Build history of the part. All positions in model axes, mm. A direction names the side the tool comes from. Round coordinates to 2 decimals unless told otherwise and drop trailing zeros. Loops run counter-clockwise (first coordinate to the right, second up) from the corner with the lowest first, then second, coordinate; pieces in that order, holes last.
from build123d import *

# Parameters (mm, degrees)
F0_R      = 20
F1_DEPTH  = 4
F2_R      = 9
F2_R_2    = 5.1
F3_DEPTH  = 20
F5_DEPTH  = 10
F6_W      = 5.5
F6_H      = 1.8
F7_DEPTH  = 5.5
F8_R      = 1.5
F9_DEPTH  = 11
F10_SIZE  = 5.99999
F12_DEPTH = 25


# Not quite as in the source:
# - a fillet or chamfer is up to 0.001 mm smaller than in the source, because OpenCascade refuses the exact size


with BuildPart() as f1:
    # F0 (on Top) → F1 (new body)
    with BuildSketch(Plane.XY):
        Circle(F0_R)
    extrude(amount=F1_DEPTH)

    # F2 (on face) → F3 (join)
    with BuildSketch(Plane.XY.offset(4)):
        Circle(F2_R)
        Circle(F2_R_2, mode=Mode.SUBTRACT)
    extrude(amount=F3_DEPTH)

    # F4 (on face) → F5 (join)
    with BuildSketch(Plane.XY.offset(4)):
        with BuildLine():
            Line((-3.5, 15), (-3.5, 8.2915619759))
            ThreePointArc((-3.5, 8.2915619759), (0, 9), (3.5, 8.2915619759))
            Line((3.5, 8.2915619759), (3.5, 15))
            Line((3.5, 15), (-3.5, 15))
        make_face()
        with BuildLine():
            Line((15, 3.5), (8.2915619759, 3.5))
            ThreePointArc((8.2915619759, 3.5), (8.8211126788, 1.785489039), (9, 0))
            ThreePointArc((9, 0), (8.8211126788, -1.785489039), (8.2915619759, -3.5))
            Line((8.2915619759, -3.5), (15, -3.5))
            Line((15, -3.5), (15, 3.5))
        make_face()
        with BuildLine():
            Line((-8.2915619759, 3.5), (-15, 3.5))
            Line((-15, 3.5), (-15, -3.5))
            Line((-15, -3.5), (-8.2915619759, -3.5))
            ThreePointArc((-8.2915619759, -3.5), (-9, 0), (-8.2915619759, 3.5))
        make_face()
        with BuildLine():
            ThreePointArc((3.5, -8.2915619759), (0, -9), (-3.5, -8.2915619759))
            Line((-3.5, -8.2915619759), (-3.5, -15))
            Line((-3.5, -15), (3.5, -15))
            Line((3.5, -15), (3.5, -8.2915619759))
        make_face()
    extrude(amount=F5_DEPTH)

    # F6 (on face) → F7 (cut)
    with BuildSketch(Plane.XY.offset(14)):
        with Locations((0, -11.6)):
            Rectangle(F6_W, F6_H)
    extrude(amount=-F7_DEPTH, mode=Mode.SUBTRACT)

    # F8 (on face) → F9 (cut)
    with BuildSketch(Plane.XZ.offset(15)):
        with Locations((0, 11.25)):
            Circle(F8_R)
    extrude(amount=-F9_DEPTH, mode=Mode.SUBTRACT)

    # F10 (size 6 in the source; OpenCascade refuses exactly that, so slightly less here)
    f10_edges = [f1.edges().sort_by_distance(p)[0] for p in [
        (15, 0, 14),
        (0, 15, 14),
        (-15, 0, 14),
    ]]
    chamfer(f10_edges, length=F10_SIZE)

    # F11 (on face) → F12 (cut)
    with BuildSketch(Plane(origin=(0, 0, 0), x_dir=(1, 0, 0), z_dir=(0, 0, -1))):
        with BuildLine():
            ThreePointArc((-10.6066017178, 10.6066017178), (-9.8758984631, 11.2901120254), (-9.1012534477, 11.9233881795))
            ThreePointArc((-9.1012534477, 11.9233881795), (-12.0208152802, 12.0208152802), (-11.9233881795, 9.1012534477))
            ThreePointArc((-11.9233881795, 9.1012534477), (-11.2901120254, 9.8758984631), (-10.6066017178, 10.6066017178))
        make_face()
        with BuildLine():
            Line((-10.6066017178, 10.6066017178), (-9.1923881554, 9.1923881554))
            ThreePointArc((-9.1923881554, 9.1923881554), (-8.7588426528, 9.8412348531), (-8.6066017178, 10.6066017178))
            ThreePointArc((-8.6066017178, 10.6066017178), (-8.7343441847, 11.3099165335), (-9.1012534477, 11.9233881795))
            ThreePointArc((-9.1012534477, 11.9233881795), (-9.8758984631, 11.2901120254), (-10.6066017178, 10.6066017178))
        make_face()
        with BuildLine():
            ThreePointArc((-11.9233881795, 9.1012534477), (-10.5398979419, 8.6077143757), (-9.1923881554, 9.1923881554))
            Line((-9.1923881554, 9.1923881554), (-10.6066017178, 10.6066017178))
            ThreePointArc((-10.6066017178, 10.6066017178), (-11.2901120254, 9.8758984631), (-11.9233881795, 9.1012534477))
        make_face()
        with BuildLine():
            ThreePointArc((9.1923881554, 9.1923881554), (10.5398979419, 8.6077143757), (11.9233881795, 9.1012534477))
            ThreePointArc((11.9233881795, 9.1012534477), (11.2901120254, 9.8758984631), (10.6066017178, 10.6066017178))
            Line((10.6066017178, 10.6066017178), (9.1923881554, 9.1923881554))
        make_face()
        with BuildLine():
            ThreePointArc((10.6066017178, 10.6066017178), (11.2901120254, 9.8758984631), (11.9233881795, 9.1012534477))
            ThreePointArc((11.9233881795, 9.1012534477), (12.427806391, 9.7800343955), (12.6066017178, 10.6066017178))
            ThreePointArc((12.6066017178, 10.6066017178), (11.3099165335, 12.4788592508), (9.1012534477, 11.9233881795))
            ThreePointArc((9.1012534477, 11.9233881795), (9.8758984631, 11.2901120254), (10.6066017178, 10.6066017178))
        make_face()
        with BuildLine():
            Line((9.1923881554, 9.1923881554), (10.6066017178, 10.6066017178))
            ThreePointArc((10.6066017178, 10.6066017178), (9.8758984631, 11.2901120254), (9.1012534477, 11.9233881795))
            ThreePointArc((9.1012534477, 11.9233881795), (8.6077143757, 10.5398979419), (9.1923881554, 9.1923881554))
        make_face()
        with BuildLine():
            ThreePointArc((12.6066017178, -10.6066017178), (12.427806391, -9.7800343955), (11.9233881795, -9.1012534477))
            ThreePointArc((11.9233881795, -9.1012534477), (11.2901120254, -9.8758984631), (10.6066017178, -10.6066017178))
            ThreePointArc((10.6066017178, -10.6066017178), (9.8758984631, -11.2901120254), (9.1012534477, -11.9233881795))
            ThreePointArc((9.1012534477, -11.9233881795), (11.3099165335, -12.4788592508), (12.6066017178, -10.6066017178))
        make_face()
        with BuildLine():
            ThreePointArc((10.6066017178, -10.6066017178), (11.2901120254, -9.8758984631), (11.9233881795, -9.1012534477))
            ThreePointArc((11.9233881795, -9.1012534477), (10.5398979419, -8.6077143757), (9.1923881554, -9.1923881554))
            Line((9.1923881554, -9.1923881554), (10.6066017178, -10.6066017178))
        make_face()
        with BuildLine():
            ThreePointArc((9.1012534477, -11.9233881795), (9.8758984631, -11.2901120254), (10.6066017178, -10.6066017178))
            Line((10.6066017178, -10.6066017178), (9.1923881554, -9.1923881554))
            ThreePointArc((9.1923881554, -9.1923881554), (8.6077143757, -10.5398979419), (9.1012534477, -11.9233881795))
        make_face()
        with BuildLine():
            ThreePointArc((-11.9233881795, -9.1012534477), (-12.0208152802, -12.0208152802), (-9.1012534477, -11.9233881795))
            ThreePointArc((-9.1012534477, -11.9233881795), (-9.8758984631, -11.2901120254), (-10.6066017178, -10.6066017178))
            ThreePointArc((-10.6066017178, -10.6066017178), (-11.2901120254, -9.8758984631), (-11.9233881795, -9.1012534477))
        make_face()
        with BuildLine():
            ThreePointArc((-8.6066017178, -10.6066017178), (-8.7588426528, -9.8412348531), (-9.1923881554, -9.1923881554))
            Line((-9.1923881554, -9.1923881554), (-10.6066017178, -10.6066017178))
            ThreePointArc((-10.6066017178, -10.6066017178), (-9.8758984631, -11.2901120254), (-9.1012534477, -11.9233881795))
            ThreePointArc((-9.1012534477, -11.9233881795), (-8.7343441847, -11.3099165335), (-8.6066017178, -10.6066017178))
        make_face()
        with BuildLine():
            Line((-10.6066017178, -10.6066017178), (-9.1923881554, -9.1923881554))
            ThreePointArc((-9.1923881554, -9.1923881554), (-10.5398979419, -8.6077143757), (-11.9233881795, -9.1012534477))
            ThreePointArc((-11.9233881795, -9.1012534477), (-11.2901120254, -9.8758984631), (-10.6066017178, -10.6066017178))
        make_face()
    extrude(amount=-F12_DEPTH, mode=Mode.SUBTRACT)


solid = f1.part
(1) Probe line 1 (Y direction, x = 0, z = 17); line 2 (Z direction, x = 0, y = -14.35); line 3 (Y direction, x = -9, z = 2.75). List the from-to ranges inside material, lowest first.
Responses:
line 1: y = -9 to -5.1, 5.1 to 9
line 2: z = 0 to 9.75, 12.75 to 14
line 3: y = -17.86 to -11.8, -9.42 to 9.42, 11.8 to 17.86
(2) Pin check, flat tips, straight feed: P1, Ø1, axis at x = 11, z = 3.5, coming from the -Y side; P2, Ø4.5, axis at x = -1, z = 12.5, coming from the -Y side; P3, Ø2, axis at x = -1.5, z = 7, coming from the +Y side. Stop position of each tip, or through.
Responses:
P1: stops at y = -17.02
P2: stops at y = -15
P3: stops at y = 15
(3) Slice it at D-D on z = 11.25. List the corners of the cut face in (x, y).
Responses:
outline: (-11.75, -3.5) - (-8.29, -3.5) arc R9 ccw to (-3.5, -8.29) - (-3.5, -15) - (-1.5, -15) - (-1.5, -12.5) - (-2.75, -12.5) - (-2.75, -10.7) - (-1.5, -10.7) - (-1.5, -4.87) arc R5.1 cw (long way) to (1.5, -4.87) - (1.5, -10.7) - (2.75, -10.7) - (2.75, -12.5) - (1.5, -12.5) - (1.5, -15) - (3.5, -15) - (3.5, -8.29) arc R9 ccw to (8.29, -3.5) - (11.75, -3.5) - (11.75, 3.5) - (8.29, 3.5) arc R9 ccw to (3.5, 8.29) - (3.5, 11.75) - (-3.5, 11.75) - (-3.5, 8.29) arc R9 ccw to (-8.29, 3.5) - (-11.75, 3.5) - close
(4) Slice it at B-B on x = 0. Count the separate pieces of the cut face and the enclosed holes in it, plus the area to 3 significant figures.
Responses:
separate pieces: 3
enclosed holes: 0
area: 384 mm2
(5) Pull direction Y, two halves, no side cores. Call faces 4 (the face through (-0.325, -13.768, 9.786)), 5 (the face through (-11, -3.5, 8)), 6 (the face through (-1.3, -10.7, 10.1)): +Y half, -Y half, draft (parallel to the pull), parting line (faces both ways), or undercut.
Responses:
face 4: draft
face 5: -Y half
face 6: undercut
(6) Slice it at A-A on z = 1.5. List the corners of the cut face in (x, y), plus the area to 3 significant figures.
Responses:
outline: circle Ø40 at (0, 0); hole circle Ø4 at (-10.61, -10.61); hole circle Ø4 at (-10.61, 10.61); hole circle Ø4 at (10.61, -10.61); hole circle Ø4 at (10.61, 10.61)
area: 1,210 mm2
(7) Which spindle directions (+Z, -Z, +X, -X, +Y, -Y) get a long thin tool onto all of the face, cutting with end or side? Do faces 1 (the face through (11, -3.5, 8)), 2 (the face through (2.74, 4.3, 13.86)), 3 (the face through (3.5, 11, 8)). Say none if no direction does.
Responses:
face 1: +Z, +X, -Y
face 2: +Z
face 3: +Z, +X, +Y
